The model under review builds one solid part; all positions refer to its coordinate system, in mm. Face numbers are marked on the shaded views. A direction names the side the tool comes from. Round coordinates to 2 decimals unless told otherwise and drop trailing zeros. Order: outer loops, then holes, each group sorted by start corner. A loop starts at its lowest first (then second) coordinate and runs counter-clockwise, first axis right, second up.
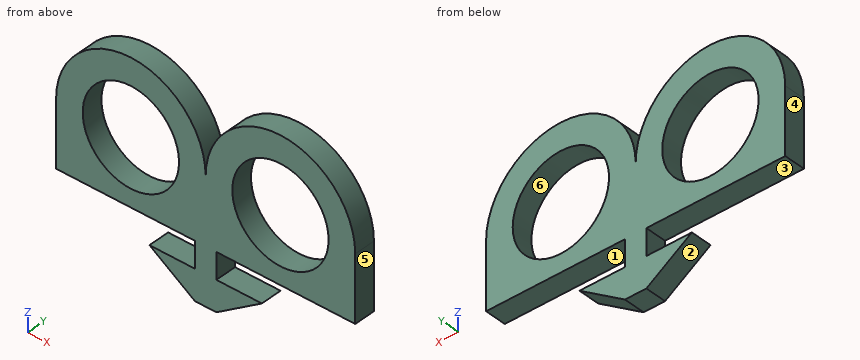
```python
from build123d import *

# Parameters (mm, degrees)
BOSS_EXTRUDE1_DEPTH = 3.5814
BOSS_EXTRUDE2_DEPTH = 3.5814
SKETCH4_R           = 8.0518
CUT_EXTRUDE2_DEPTH  = 4.5814


with BuildPart() as part:
    # Sketch1 → Boss-Extrude1 (new body)
    with BuildSketch(Plane(origin=(0, 0, 0), x_dir=(1, 0, 0), z_dir=(0, 1, 0))):
        Polygon((-25.0063, -13.1856988), (25.0063, -13.1856988), (25.0063, -2.1874988), (1.7907, -2.1874988), (1.7907, 2.1874988), (9.398, 2.1874988), (1.7907, 7.2674988), (-1.7907, 7.2674988), (-9.398, 2.1874988), (-1.7907, 2.1874988), (-1.7907, -2.1874988), (-25.0063, -2.1874988), align=None)
    extrude(amount=BOSS_EXTRUDE1_DEPTH)

    # Sketch3 → Boss-Extrude2 (add)
    with BuildSketch(Plane(origin=(0, 3.5814, 0), x_dir=(1, 0, 0), z_dir=(0, 1, 0))):
        with BuildLine():
            Line((0, -13.1856988), (-25.0063, -13.1856988))
            ThreePointArc((-25.0063, -13.1856988), (-12.50315, -25.6888488), (0, -13.1856988))
        make_face()
        with BuildLine():
            Line((25.0063, -13.1856988), (0, -13.1856988))
            ThreePointArc((0, -13.1856988), (12.50315, -25.6888488), (25.0063, -13.1856988))
        make_face()
    extrude(amount=-BOSS_EXTRUDE2_DEPTH)

    # Sketch4 → Cut-Extrude2 (cut, through all)
    with BuildSketch(Plane(origin=(0, 3.5814, 0), x_dir=(1, 0, 0), z_dir=(0, 1, 0))):
        with Locations((-12.50315, -13.1856988)):
            Circle(SKETCH4_R)
        with Locations((12.50315, -13.1856988)):
            Circle(SKETCH4_R)
    extrude(amount=-CUT_EXTRUDE2_DEPTH, mode=Mode.SUBTRACT)


solid = part.part
```
(1) Insertion check: pin 1 (1.1 mm diameter, centred on x = -14, y = 1, fed in from -Z); pin 2 (9.5 mm diameter, centred on x = -12.5, z = 13.19, fed in from +Y); pin 3 (1.1 mm diameter, centred on y = 2, z = 1, fed in from -X); pin 4 (1.1 mm diameter, centred on x = 5, y = 2.5, fed in from +Z). Each pin has a flat end and moves straight along its axis. Give the tip position at first contact, or say it passes through.
Data:
pin 1: stops at z = 2.19
pin 2: passes through
pin 3: stops at x = -1.79
pin 4: stops at z = 23.58
(2) For the marked faces 1, 2 and 3, list the 3-axis set-ups (+Z, -Z, +X, -X, +Y, -Y) from which the entire face can be reached by the end or side of a thin tool; tool diameter is ignored.
Data:
face 1: +X, +Y, -Y
face 2: -Z, -X, +Y, -Y
face 3: -X, +Y, -Y
(3) Draft analysis for pull direction X (two halves, no side actions). For the marked faces 4, 5 and 6, state which applies: pulls with the +X half, pulls with the -X half, needs draft (parallel to the pull), parting line crosses it, or undercut.
Data:
face 4: pulls with the -X half
face 5: pulls with the +X half
face 6: undercut
(4) Consider section C-C (x = 17.5). Write out the cut boundary in (y, z), and give its area (3 significant figures).
Data:
outline: (0, 2.19) - (3.58, 2.19) - (3.58, 6.87) - (0, 6.87) - close; (0, 19.5) - (3.58, 19.5) - (3.58, 24.65) - (0, 24.65) - close
area: 35.2 mm2
(5) Consider section D-D (z = 23). Write out the cut boundary in (x, y), and give its area (3 significant figures).
Data:
outline: (-20.25, 0) - (-4.76, 0) - (-4.76, 3.58) - (-20.25, 3.58) - close; (4.76, 0) - (20.25, 0) - (20.25, 3.58) - (4.76, 3.58) - close
area: 111 mm2
(6) Consider section A-A (z = 14). Write out the cut boundary in (x, y), and give its area (3 significant figures).
Data:
outline: (-24.98, 0) - (-20.51, 0) - (-20.51, 3.58) - (-24.98, 3.58) - close; (-4.49, 0) - (-0.03, 0) - (-0.03, 3.58) - (-4.49, 3.58) - close; (0.03, 0) - (4.49, 0) - (4.49, 3.58) - (0.03, 3.58) - close; (20.51, 0) - (24.98, 0) - (24.98, 3.58) - (20.51, 3.58) - close
area: 64.0 mm2
(7) Consider section B-B (y = 0.75). Write out the cut boundary in (x, z).
Data:
outline: (-25.01, 2.19) - (-1.79, 2.19) - (-1.79, -2.19) - (-9.4, -2.19) - (-1.79, -7.27) - (1.79, -7.27) - (9.4, -2.19) - (1.79, -2.19) - (1.79, 2.19) - (25.01, 2.19) - (25.01, 13.19) arc R12.5 ccw to (0, 13.19) arc R12.5 ccw to (-25.01, 13.19) - close; hole circle Ø16.1 at (-12.5, 13.19); hole circle Ø16.1 at (12.5, 13.19)
(8) To check wall thickness, follow probe 1 along X at (y, z) = (0.75, 7); probe 2 along X at (y, z) = (2.3, 15); probe 3 along Z at (x, y) = (6, 0.8). State the ranges of each line that lie inside material, in increasing order.
Data:
probe 1: x = -25.01 to -17.66, -7.35 to 7.35, 17.66 to 25.01
probe 2: x = -24.87 to -20.35, -4.66 to -0.13, 0.13 to 4.66, 20.35 to 24.87
probe 3: z = -4.46 to -2.19, 2.19 to 8.44, 17.93 to 23.86
